Autodesk Fusion 360 part; units mm, degrees
sketch "Sketch1" plane through (0, 0, 0) normal (0, 0, 1) x (1, 0, 0)
  line L0 (15, -15) -> (-15, -15)
  line L1 (-15, -15) -> (-15, 15)
  line L2 (-15, 15) -> (15, 15)
  line L3 (15, 15) -> (15, -15)
  line L4 (15, -15) -> (-15, 15) construction
  line L5 (-15, -15) -> (15, 15) construction
  dimension "d1" = 30
  dimension "d2" = 30
extrude "Extrude1" add sketch "Sketch1" along normal blind 2 makes body 1
sketch "Sketch2" plane through (0, 0, 2) normal (0, 0, 1) x (-1, 0, 0)
  line L0 (-15, -15) -> (15, -15)
  line L1 (15, -15) -> (15, 15)
  line L2 (15, 15) -> (-15, 15)
  line L3 (-15, 15) -> (-15, -15)
  line L4 (15, 15) -> (10, 15) construction
  line L5 (10, 15) -> (10, 10) construction
  line L6 (10, 10) -> (15, 10) construction
  line L7 (15, 10) -> (15, 15) construction
  line L8 (-15, 15) -> (-10, 15) construction
  line L9 (-10, 15) -> (-10, 10) construction
  line L10 (-10, 10) -> (-15, 10) construction
  line L11 (-15, 10) -> (-15, 15) construction
  line L12 (10, 15) -> (-10, 15)
  line L13 (-10, 15) -> (-10, 10)
  line L14 (-10, 10) -> (10, 10)
  line L15 (10, 10) -> (10, 15)
  dimension "d5" = 5
  dimension "d6" = 5
  dimension "d7" = 5
  dimension "d8" = 5
extrude "Extrude2" add sketch "Sketch2" along normal blind 40 contours L2 L12 L13 L14 L15 bodies 1
sketch "Sketch3" plane through (0, -15, 0) normal (0, -1, 0) x (1, 0, 0)
  line L0 (-15, 0) -> (15, 0)
  line L1 (15, 0) -> (15, 2)
  line L2 (15, 2) -> (10, 2)
  line L3 (10, 2) -> (10, 42)
  line L4 (10, 42) -> (-10, 42)
  line L5 (-10, 42) -> (-10, 2)
  line L6 (-10, 2) -> (-15, 2)
  line L7 (-15, 2) -> (-15, 0)
  line L8 (10, 2) -> (0, 2) construction
  line L9 (0, 2) -> (0, 27) construction
  line L10 (0, 27) -> (10, 27) construction
  line L11 (10, 27) -> (10, 2) construction
  circle A0 centre (0, 27) radius 2.55
  dimension "d11" = 10
  dimension "d12" = 25
  dimension "d13" = 5.1
sketch "Sketch4" plane through (0, -15, 0) normal (0, -1, 0) x (1, 0, 0)
  line L0 (-15, 0) -> (15, 0)
  line L1 (15, 0) -> (15, 2)
  line L2 (15, 2) -> (10, 2)
  line L3 (10, 2) -> (10, 42)
  line L4 (10, 42) -> (-10, 42)
  line L5 (-10, 42) -> (-10, 2)
  line L6 (-10, 2) -> (-15, 2)
  line L7 (-15, 2) -> (-15, 0)
  line L8 (0, 27) -> (1.75, 27) construction
  line L9 (0, 27) -> (-1.75, 27) construction
  circle A0 centre (1.75, 27) radius 0.5
  circle A1 centre (-1.75, 27) radius 0.5
  point P0 (0, 27)
  dimension "d14" = 1.75
  dimension "d15" = 1.75
  dimension "d16" = 1
  dimension "d17" = 1
extrude "Extrude3" cut sketch "Sketch4" against normal up to surface (5 mm away) contours A0 | A1 bodies 1
extrude "Extrude4" cut sketch "Sketch3" against normal blind 3 contours A0 bodies 1
copy_body "Body->Comp1" bodies 1 removing the originals makes body 2 in component "Detector_Holder"
component "Detector_Holder" placed x (1, 0, 0) y (0, 1, 0) z (0, 0, 1) at (0, 0, 0)
Geometry: final body of the model. Coordinates: model frame, mm. A direction names the side the tool comes from. Round coordinates to 2 decimals unless told otherwise and drop trailing zeros. Write each loop counter-clockwise with the first axis right and the second up, starting at its lowest first coordinate (ties: lowest second). Pieces come first, ordered by that corner, then holes. Notation, with made-up numbers: M 83,85.5 L 136,85.5 A27 ccw 136,108.5 Z; hole C -28,4 d10. An arc over 180 degrees is marked long. Answer in a Markdown table with one row per item. Add a question column.
(1) Cut plane D-D, the plane z = 12. Return the cut outline in (x, y), then the cut area to 3 significant figures.
(2) Cut plane B-B, the plane x = -1.75. Return the cut outline in (y, z), then the cut area to 3 significant figures.
(3) Cut plane A-A, the plane z = 27. Return the cut outline in (x, y), then the cut area to 3 significant figures.
(4) Contact query for flat-ended pins moving along their axis: pin 1 (6.5 mm diameter, centred on x = 0, z = 27, fed in from +Y); pin 2 (1 mm diameter, centred on x = 7.5, y = -2, fed in from +Z); pin 3 (4 mm diameter, centred on y = -12.5, z = 19.5, fed in from +X); pin 4 (5.5 mm diameter, centred on x = 1, z = 27.5, fed in from -Y). Output: stop coordinate, or through.
(5) Reachability of faces 1 (the face through (0, -10, 22)), 2 (the face through (10, -13, 22)), 3 (the face through (-0.33, -13.52, 29.53)) from +Z, -Z, +X, -X, +Y, -Y: full face, straight path, thin tool, end or side. Return the list, or none.
(6) Ray query, L1, parallel to Z at x = -1.75, y = -11.35; L2, parallel to Y at x = 0, z = 36.5; L3, parallel to Z at x = -5.75, y = 9.5. Return the intervals inside material, ascending.
(7) Cut plane C-C, the plane x = -8. Return the cut outline in (y, z).
(8) Draft query along X for faces 4 (the face through (-3, -15, 21)), 5 (the face through (0, -12, 27)), 6 (the face through (-10, -12, 22)). Return one class per face: pulls with the +X half, pulls with the -X half, needs draft (parallel to the pull), parting line crosses it, or undercut.
Established:
| question | item | result |
|---|---|---|
| 1 | outline | M -10,-15 L 10,-15 L 10,-10 L -10,-10 Z |
| 1 | area | 100 mm² |
| 2 | outline | M -15,0 L 15,0 L 15,2 L -10,2 L -10,26.5 L -12,26.5 L -12,25.15 L -15,25.15 Z; M -15,28.85 L -12,28.85 L -12,27.5 L -10,27.5 L -10,42 L -15,42 Z |
| 2 | area | 247 mm² |
| 3 | outline | M -10,-15 L -2.55,-15 L -2.55,-12 L -2.25,-12 L -2.25,-10 L -10,-10 Z; M -1.25,-12 L 1.25,-12 L 1.25,-10 L -1.25,-10 Z; M 2.25,-12 L 2.55,-12 L 2.55,-15 L 10,-15 L 10,-10 L 2.25,-10 Z |
| 3 | area | 80.7 mm² |
| 4 | pin 1 | y = -10 |
| 4 | pin 2 | z = 2 |
| 4 | pin 3 | x = 10 |
| 4 | pin 4 | y = -15 |
| 5 | face 1 | +Z, +X, -X, +Y |
| 5 | face 2 | +Z, +X, +Y, -Y |
| 5 | face 3 | -Y |
| 6 | L1 | 0 to 26.5, 27.5 to 42 |
| 6 | L2 | -15 to -10 |
| 6 | L3 | 0 to 2 |
| 7 | outline | M -15,0 L 15,0 L 15,2 L -10,2 L -10,42 L -15,42 Z |
| 8 | face 4 | needs draft |
| 8 | face 5 | undercut |
| 8 | face 6 | pulls with the -X half |
